Check sheet for the modelled part. Datum: model origin and axes. Units: mm. A direction names the side the tool comes from. Round coordinates to 2 decimals unless told otherwise and drop trailing zeros. Loops run counter-clockwise (first coordinate to the right, second up) from the corner with the lowest first, then second, coordinate; pieces in that order, holes last. Notation, with made-up numbers: (26, 48) -> (60, 48) arc R16 ccw to (60, 59) -> close; hole circle Ø3 at (75, 38.5). An arc over 180 degrees is marked (long way). Return JSON: item names as keys, results as strings.
Autodesk Inventor part; units mm, degrees
ref_plane "YZ Plane" through (0, 0, 0) normal (1, 0, 0) x (0, 1, 0)
ref_plane "XZ Plane" through (0, 0, 0) normal (0, 1, 0) x (-1, 0, 0)
ref_plane "XY Plane" through (0, 0, 0) normal (0, 0, 1) x (1, 0, 0)
sketch "Boceto1" plane through (0, 0, 0) normal (0, 1, 0) x (-1, 0, 0)
  line L0 (0, 145) -> (24.25, 145)
  line L1 (145, 24.25) -> (145, -24.25)
  line L2 (145, 24.25) -> (24.25, 145)
  line L3 (24.25, -145) -> (145, -24.25)
  line L4 (24.25, -145) -> (0, -145)
  circle A0 centre (29.25, -122) radius 2
  circle A1 centre (122, -29.25) radius 2
  circle A2 centre (122, 29.25) radius 2
  circle A3 centre (29.25, 122) radius 2
  line L5 (0, -145) -> (0, 145)
  point P0 (0, 0)
  dimension "d13" = 4
  dimension "d16" = 4
  dimension "d18" = 4
  dimension "d20" = 4
extrude "Extrusión1" add sketch "Boceto1" along normal blind 3
sketch "Boceto2" plane through (0, 3, 0) normal (0, 1, 0) x (1, 0, 0)
  line L0 (21.25, -21.25) -> (21.25, 21.25)
  line L1 (21.25, 21.25) -> (-21.25, 21.25)
  line L2 (-21.25, 21.25) -> (-21.25, -21.25)
  line L3 (-24.25, 24.25) -> (24.25, 24.25)
  line L4 (24.25, 24.25) -> (24.25, -24.25)
  line L5 (-24.25, -24.25) -> (-24.25, 24.25)
  line L6 (8.5, -21.25) -> (8.5, -24.25)
  line L7 (-8.5, -24.25) -> (-8.5, -21.25)
  line L8 (-21.25, -21.25) -> (-8.5, -21.25)
  line L9 (8.5, -21.25) -> (21.25, -21.25)
  line L10 (24.25, -24.25) -> (8.5, -24.25)
  line L11 (-8.5, -24.25) -> (-24.25, -24.25)
  dimension "d29" = 42.5
  dimension "d30" = 42.5
  dimension "d31" = 48.5
  dimension "d32" = 48.5
extrude "Extrusión2" add sketch "Boceto2" along normal blind 44
sketch "Boceto3" plane through (0, 3, 0) normal (0, 1, 0) x (1, 0, 0)
  line L0 (-21.25, 21.25) -> (-21.25, -21.25)
  line L1 (21.25, 21.25) -> (21.25, -21.25)
  line L2 (-21.25, 21.25) -> (21.25, 21.25)
  line L3 (21.25, 21.25) -> (21.25, -21.25)
  line L4 (21.25, -21.25) -> (-21.25, -21.25)
  line L5 (-21.25, -21.25) -> (-21.25, 21.25)
extrude "Extrusión3" add sketch "Boceto3" along normal blind 4
sketch "Boceto5" plane through (0, 3, 0) normal (0, 1, 0) x (1, 0, 0)
  line L0 (-142, 9) -> (-130, 9)
  line L1 (-130, 9) -> (-130, -9)
  line L2 (-130, -9) -> (-142, -9)
  line L3 (-9, -130) -> (-9, -142)
  line L4 (-9, 130) -> (-9, 142)
  line L5 (-142, 9) -> (-142, -9)
  line L6 (-9, -130) -> (0, -130)
  line L7 (-9, -142) -> (0, -142)
  line L8 (0, -130) -> (0, -142)
  line L9 (0, -145) -> (0, 145)
  line L10 (-9, 142) -> (0, 142)
  line L11 (0, 130) -> (0, 142)
  line L12 (-9, 130) -> (0, 130)
  line L13 (-8.5, -21.25) -> (-8.5, -33.25)
  line L14 (-8.5, -33.25) -> (0, -33.25)
  line L15 (0, -21.25) -> (0, -33.25)
  dimension "d72" = 12
extrude "Extrusión5" cut sketch "Boceto5" against normal blind 3
sketch "Boceto8" plane through (0, 3, 0) normal (0, -1, 0) x (1, 0, 0)
  line L0 (24.25, -24.25) -> (-24.25, -24.25)
  line L1 (8.5, 24.25) -> (24.25, 24.25)
  line L2 (0, -24.25) -> (24.25, -24.25)
  line L3 (24.25, -24.25) -> (24.25, 24.25)
  line L4 (24.25, 24.25) -> (0, 24.25)
  line L5 (0, 24.25) -> (0, -24.25)
  point P0 (0, 0)
extrude "Extrusión8" add sketch "Boceto8" along normal blind 3
sketch "Boceto9" plane through (-8.5, 3, 21.25) normal (0, 0, 1) x (1, 0, 0)
  line L0 (0, 0) -> (0, 4)
  line L1 (17, 0) -> (0, 0)
  line L2 (0, 4) -> (17, 4)
  line L3 (17, 4) -> (17, 0)
  line L4 (17, 0) -> (0, 0)
  line L5 (0, 0) -> (0, 4)
  point P0 (8.5, -3)
extrude "Extrusión9" add sketch "Boceto9" along normal blind 3
properties part number "Base Definitiva" material "Plástico ABS"
Q1. Section check D-D (z = -67). Record the boundary of the cut face in (x, y).
Results list:
{"outline": "(-102.25, 0) -> (0, 0) -> (0, 3) -> (-102.25, 3) -> close"}
Q2. Go/stop test with flat-tipped pins: pin 1 (3.5 mm diameter, centred on y = 1.5, z = 144, fed in from +X); pin 2 (6 mm diameter, centred on x = -110.5, z = 60.5, fed in from +Y); pin 3 (2.5 mm diameter, centred on x = -138, y = 1, fed in from -Z). Record where each tip stops, or that it passes through.
Results list:
{"pin 1": "x = 0", "pin 2": "y = 3", "pin 3": "z = -32.5"}
Q3. Section check C-C (z = 16). Record the boundary of the cut face in (x, y).
Results list:
{"outline": "(-145, 0) -> (24.25, 0) -> (24.25, 47) -> (21.25, 47) -> (21.25, 7) -> (-21.25, 7) -> (-21.25, 47) -> (-24.25, 47) -> (-24.25, 3) -> (-145, 3) -> close"}
Q4. Draft check along Z on faces 1 (the flat face through (21.25, 27, 0)), 2 (the flat face through (24.25, 24, 0)), 3 (the flat face through (-85.47, 1.48, 83.78)). Enter one of: released by +Z, released by -Z, zero draft, split by the parting line, or undercut.
Results list:
{"face 1": "undercut", "face 2": "zero draft", "face 3": "released by +Z"}
Q5. Section check B-B (x = -18.5). Record the boundary of the cut face in (y, z), then the cut area to 3 significant figures.
Results list:
{"outline": "(0, -145) -> (3, -145) -> (3, -24.25) -> (47, -24.25) -> (47, -21.25) -> (7, -21.25) -> (7, 21.25) -> (47, 21.25) -> (47, 24.25) -> (3, 24.25) -> (3, 145) -> (0, 145) -> close", "area": "1,300 mm^2"}
Q6. Tool access check on faces 4 (the flat face through (-24.25, 25, 0)), 5 (the flat face through (-21.25, 27, 0)), 6 (the flat face through (0, 47, -23)). Record the directions out of +Z, -Z, +X, -X, +Y, -Y that give a thin tool (end or side, any length) a straight path to the whole face; none if there is none.
Results list:
{"face 4": "+Z, -Z, -X, +Y", "face 5": "+Y", "face 6": "+Z, -Z, +X, -X, +Y"}
Q7. Section check A-A (y = 19). Record the boundary of the cut face in (x, z).
Results list:
{"outline": "(-24.25, -24.25) -> (24.25, -24.25) -> (24.25, 24.25) -> (8.5, 24.25) -> (8.5, 21.25) -> (21.25, 21.25) -> (21.25, -21.25) -> (-21.25, -21.25) -> (-21.25, 21.25) -> (-8.5, 21.25) -> (-8.5, 24.25) -> (-24.25, 24.25) -> close"}
Q8. Material ranges on line 1 (Z direction, x = -20, y = 43.5); line 2 (Z direction, x = -122, y = 2); line 3 (Z direction, x = -2, y = 40), recorded low to high.
Results list:
{"line 1": "-24.25 to -21.25, 21.25 to 24.25", "line 2": "-47.25 to -31.25, -27.25 to 27.25, 31.25 to 47.25", "line 3": "-24.25 to -21.25"}
